Source: CAD feature listing. Evaluate the final solid. Frame: model axes, mm. Face numbers are marked on the shaded views. A direction names the side the tool comes from. Round coordinates to 2 decimals unless told otherwise and drop trailing zeros. Write each loop counter-clockwise with the first axis right and the second up, starting at its lowest first coordinate (ties: lowest second). Pieces come first, ordered by that corner, then holes. Notation, with made-up numbers: M -13.5,83.5 L 4.5,83.5 A33 cw 4.5,122.5 Z; hole C -3.75,31 d4. An arc over 180 degrees is marked long. Answer in a Markdown table with one row per item. Add a question column.
Item 1: Contact query for flat-ended pins moving along their axis: pin 1 (1 mm diameter, centred on x = 0, z = 4.5, fed in from -Y); pin 2 (8 mm diameter, centred on y = -15, z = 8.5, fed in from +X); pin 3 (4.5 mm diameter, centred on x = 0, y = 0, fed in from +Z); pin 4 (7 mm diameter, centred on x = 3, z = 11.5, fed in from -Y). Output: stop coordinate, or through.
Item 2: Cut plane D-D on y = -6.5. Return loops of the section in (x, z), and give its area (4 significant figures).
Item 3: Cut plane A-A on x = 0. Return loops of the section in (y, z), and give its area (3 significant figures).
Item 4: Set-up query: the marked faces 4, 5 and 6. Return all of +Z, -Z, +X, -X, +Y, -Y with unobstructed straight access to the full face (end or side cutting, diameter ignored); none if empty.
Item 5: Material intervals for probe 1 along Y at (x, z) = (-1.5, 6.75); probe 2 along X at (y, z) = (-7.75, 16.75); probe 3 along Y at (x, z) = (0, 3.6), sorted ascending.
Item 6: Cut plane C-C on z = 16.75. Return loops of the section in (x, y).
Item 7: Cut plane B-B on y = 0. Return loops of the section in (x, z).
Item 8: Mould query, pull axis Y, two halves, no side actions, for the marked faces 1, 2 and 3. Classes: released by +Y, released by -Y, zero draft, split by the parting line, or undercut.
from build123d import *

# Parameters (mm, degrees)
F0_R     = 2.5
F1_DEPTH = 5
F3_DEPTH = 14.5
F4_R     = 2
F5_DEPTH = 14.5
F6_R     = 1
F7_R     = 1
F8_R     = 2


with BuildPart() as f1:
    # F0 (on Top) → F1 (new body)
    with BuildSketch(Plane.XY):
        Polygon((-9, 9), (-9, -21), (21, 9), align=None)
        Circle(F0_R, mode=Mode.SUBTRACT)
    extrude(amount=F1_DEPTH)

    # F2 (on face) → F3 (join)
    with BuildSketch(Plane.XY.offset(5)):
        Polygon((-9, 9), (-9, -21), (-5, -17), (-5, 5), (17, 5), (21, 9), align=None)
    extrude(amount=F3_DEPTH)

    # F4 (on face) → F5 (cut, through all)
    with BuildSketch(Plane.XY.offset(19.5)):
        with Locations((-3.93934, 3.93934)):
            Circle(F4_R)
    extrude(amount=-F5_DEPTH, mode=Mode.SUBTRACT)

    # F6
    f6_edges = [f1.edges().sort_by_distance(p)[0] for p in [
        (21, 9, 9.75),
    ]]
    fillet(f6_edges, radius=F6_R)

    # F7
    f7_edges = [f1.edges().sort_by_distance(p)[0] for p in [
        (-9, -21, 9.75),
    ]]
    fillet(f7_edges, radius=F7_R)

    # F8
    f8_edges = [f1.edges().sort_by_distance(p)[0] for p in [
        (-9, 9, 9.75),
    ]]
    fillet(f8_edges, radius=F8_R)


solid = f1.part
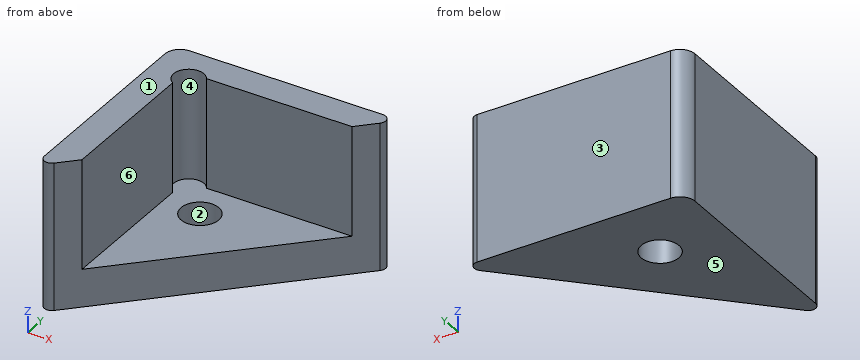
Results below:
| question | item | result |
|---|---|---|
| 1 | pin 1 | y = -12.5 |
| 1 | pin 2 | x = -1.06 |
| 1 | pin 3 | through |
| 1 | pin 4 | y = 5 |
| 2 | outline | M -9,0 L 5.5,0 L 5.5,5 L -5,5 L -5,19.5 L -9,19.5 Z |
| 2 | area | 130.5 mm2 |
| 3 | outline | M -12,0 L -2.5,0 L -2.5,5 L -12,5 Z; M 2.5,0 L 9,0 L 9,19.5 L 5,19.5 L 5,5 L 2.5,5 Z |
| 3 | area | 138 mm2 |
| 4 | face 4 | +Z |
| 4 | face 5 | -Z, +X, -X, +Y, -Y |
| 4 | face 6 | +Z, +X, -Y |
| 5 | probe 1 | 5 to 9 |
| 5 | probe 2 | -9 to -5 |
| 5 | probe 3 | -12 to -2.5, 2.5 to 9 |
| 6 | outline | M -9,-18.59 A1 ccw -7.29,-19.29 L -5,-17 L -5,2.24 A2 cw long -2.24,5 L 17,5 L 19.29,7.29 A1 ccw 18.59,9 L -7,9 A2 ccw -9,7 Z |
| 7 | outline | M -9,0 L -2.5,0 L -2.5,5 L -5,5 L -5,19.5 L -9,19.5 Z; M 2.5,0 L 12,0 L 12,5 L 2.5,5 Z |
| 8 | face 1 | zero draft |
| 8 | face 2 | undercut |
| 8 | face 3 | released by +Y |
